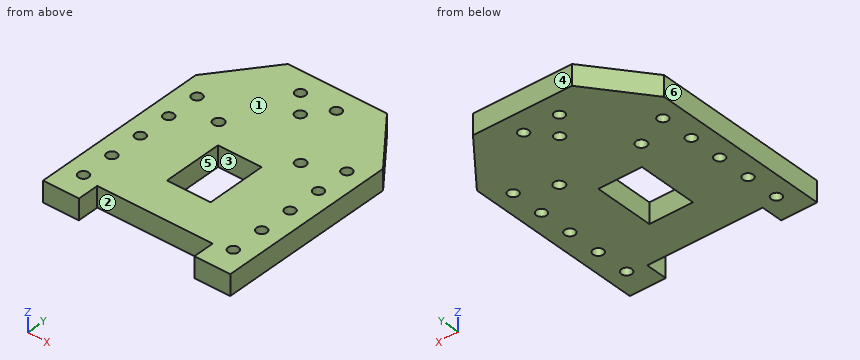
from build123d import *

# Parameters (mm, degrees)
ESBO_O1_R                = 2
ESBO_O1_R_2              = 2.086716092
ESBO_O1_R_3              = 2.086717953
RESSALTO_EXTRUS_O1_DEPTH = 8
ESBO_O2_R                = 2
CORTE_EXTRUS_O1_DEPTH    = 9


with BuildPart() as part:
    # Esboço1 → Ressalto-extrusão1 (new body)
    with BuildSketch(Plane.XY):
        Polygon((19.311716217, 92), (-19.311716217, 92), (-36.5, 70), (-36.5, 0), (-22.499999998, 0), (-22.499999998, 8.400000004), (22.499999998, 8.400000004), (22.499999998, 0), (36.5, 0), (36.5, 70), align=None)
        with Locations((0, 75)):
            Circle(ESBO_O1_R, mode=Mode.SUBTRACT)
        with Locations((-7, 83.3)):
            Circle(ESBO_O1_R, mode=Mode.SUBTRACT)
        with Locations((7, 83.3)):
            Circle(ESBO_O1_R, mode=Mode.SUBTRACT)
        with Locations((-29.2, 10)):
            Circle(ESBO_O1_R, mode=Mode.SUBTRACT)
        with Locations((29.2, 10)):
            Circle(ESBO_O1_R, mode=Mode.SUBTRACT)
        with Locations((-16, 56.354540575)):
            Circle(ESBO_O1_R_2, mode=Mode.SUBTRACT)
        with Locations((16, 56.354540575)):
            Circle(ESBO_O1_R_3, mode=Mode.SUBTRACT)
        Polygon((0, 47.257129716), (8.5, 47.257129716), (8.5, 23.917682695), (0, 23.917682695), (-8.5, 23.917682695), (-8.5, 47.257129716), align=None, mode=Mode.SUBTRACT)
    extrude(amount=RESSALTO_EXTRUS_O1_DEPTH)

    # Esboço2 → Corte-extrusão1 (cut, through all)
    with BuildSketch(Plane(origin=(0, 0, 0), x_dir=(-1, 0, 0), z_dir=(0, 0, -1))):
        with Locations((29.2, 23)):
            Circle(ESBO_O2_R)
        with Locations((29.2, 36)):
            Circle(ESBO_O2_R)
        with Locations((29.2, 49)):
            Circle(ESBO_O2_R)
        with Locations((29.2, 62)):
            Circle(ESBO_O2_R)
        with Locations((-29.2, 49)):
            Circle(ESBO_O2_R)
        with Locations((-29.2, 36)):
            Circle(ESBO_O2_R)
        with Locations((-29.2, 62)):
            Circle(ESBO_O2_R)
        with Locations((-29.2, 23)):
            Circle(ESBO_O2_R)
    extrude(amount=-CORTE_EXTRUS_O1_DEPTH, mode=Mode.SUBTRACT)


solid = part.part
For this review, take the finished solid that the model builds, in its own axes (mm). Face numbers are marked on the shaded views. A direction names the side the tool comes from. Coordinates: 2 decimals unless noted, no trailing zeros. Loops run counter-clockwise (first coordinate to the right, second up) from the corner with the lowest first, then second, coordinate; pieces in that order, holes last. Notation, with made-up numbers: (-22, -6.75) - (-16, -6.75) arc R29 cw to (-16, 23.25) - close; hole circle Ø11 at (-22.75, 7.5). An arc over 180 degrees is marked (long way). Return JSON: item names as keys, results as strings.
Item 1: For line 1 (Y direction, x = 0, z = 6.5); line 2 (Y direction, x = 7, z = 3.5); line 3 (X direction, y = 56.5, z = 2.5), list the stretches that pass through material, from the lowest coordinate up.
Determined:
{"line 1": "y = 8.4 to 23.92, 47.26 to 73, 77 to 92", "line 2": "y = 8.4 to 23.92, 47.26 to 81.3, 85.3 to 92", "line 3": "x = -36.5 to -18.08, -13.92 to 13.92, 18.08 to 36.5"}
Item 2: Take a section at D-D (z = 1). State how many separate pieces and enclosed holes the cut face has, then the cut area to 3 significant figures.
Determined:
{"separate pieces": "1", "enclosed holes": "16", "area": "5,370 mm2"}
Item 3: For the marked faces 1, 2 and 3, list the 3-axis set-ups (+Z, -Z, +X, -X, +Y, -Y) from which the entire face can be reached by the end or side of a thin tool; tool diameter is ignored.
Determined:
{"face 1": "+Z, +X, -X, +Y, -Y", "face 2": "+Z, -Z, -Y", "face 3": "+Z, -Z"}
Item 4: Insertion check: pin 1 (2.5 mm diameter, centred on x = -29.2, y = 10, fed in from +Z); pin 2 (2 mm diameter, centred on x = -19.5, z = 1, fed in from -Y). Each pin has a flat end and moves straight along its axis. Give the tip position at first contact, or say it passes through.
Determined:
{"pin 1": "passes through", "pin 2": "stops at y = 8.4"}
Item 5: Take a section at A-A (y = 42). Give the boundary of the cut face in (x, z), then the cut area to 3 significant figures.
Determined:
{"outline": "(-36.5, 0) - (-8.5, 0) - (-8.5, 8) - (-36.5, 8) - close; (8.5, 0) - (36.5, 0) - (36.5, 8) - (8.5, 8) - close", "area": "448 mm2"}
Item 6: Mouldability with a two-part tool opening along X and no side actions: class the marked faces 4, 5 and 6 as pulls with the +X half, pulls with the -X half, needs draft (parallel to the pull), parting line crosses it, or undercut.
Determined:
{"face 4": "needs draft", "face 5": "undercut", "face 6": "pulls with the -X half"}
Item 7: Take a section at C-C (y = 10). Give the boundary of the cut face in (x, z).
Determined:
{"outline": "(-36.5, 0) - (-31.2, 0) - (-31.2, 8) - (-36.5, 8) - close; (-27.2, 0) - (27.2, 0) - (27.2, 8) - (-27.2, 8) - close; (31.2, 0) - (36.5, 0) - (36.5, 8) - (31.2, 8) - close"}
Item 8: Take a section at B-B (x = 4). Give the boundary of the cut face in (y, z), then the cut area to 3 significant figures.
Determined:
{"outline": "(8.4, 0) - (23.92, 0) - (23.92, 8) - (8.4, 8) - close; (47.26, 0) - (92, 0) - (92, 8) - (47.26, 8) - close", "area": "482 mm2"}
